Could you check a few things on this model? Use its own coordinates, in mm. Face numbers are marked on the shaded views. Round coordinates to 2 decimals unless told otherwise and drop trailing zeros. Loops run counter-clockwise (first coordinate to the right, second up) from the corner with the lowest first, then second, coordinate; pieces in that order, holes last. Notation, with made-up numbers: (12.5, -7) -> (41.5, -7) arc R13 ccw to (41.5, 10) -> close; hole circle Ø7 at (55, 39). An arc over 180 degrees is marked (long way). Use CSV: the item, a comma, the result in double quotes. Start each with the question number.
```python
from build123d import *

# Parameters (mm, degrees)
F0_W     = 25.4
F0_H     = 38.1
F0_R     = 6.35
F1_DEPTH = 133.35
F2_SIZE  = 7.62
F3_SIZE  = 7.62
F4_SIZE  = 7.62
F5_SIZE  = 7.62


with BuildPart() as f1:
    # F0 (on Front) → F1 (new body, symmetric)
    with BuildSketch(Plane.XZ):
        Rectangle(F0_W, F0_H)
        with Locations((0, 9.525)):
            Circle(F0_R, mode=Mode.SUBTRACT)
    extrude(amount=F1_DEPTH, both=True)

    # F2
    f2_edges = [f1.edges().sort_by_distance(p)[0] for p in [
        (12.7, 0, 19.05),
    ]]
    chamfer(f2_edges, length=F2_SIZE)

    # F3
    f3_edges = [f1.edges().sort_by_distance(p)[0] for p in [
        (-12.7, 0, 19.05),
    ]]
    chamfer(f3_edges, length=F3_SIZE)

    # F4
    f4_edges = [f1.edges().sort_by_distance(p)[0] for p in [
        (-12.7, 0, -19.05),
    ]]
    chamfer(f4_edges, length=F4_SIZE)

    # F5
    f5_edges = [f1.edges().sort_by_distance(p)[0] for p in [
        (12.7, 0, -19.05),
    ]]
    chamfer(f5_edges, length=F5_SIZE)


solid = f1.part
```
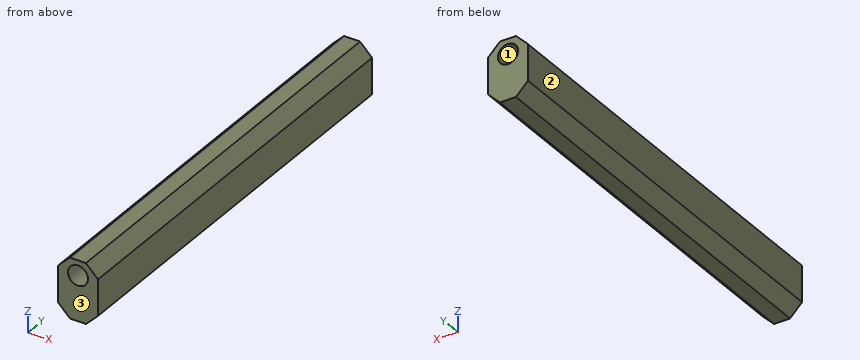
1. Suppose I cut it at D-D (z = -15). List the corners of the cut face in (x, y) for me, then the cut area to 3 significant figures.
2. Will these pins go through, and if not, where does the flat tip stop? pin 1 (8 mm diameter, centred on x = -5.5, y = 59.5, fed in from +Z); pin 2 (2 mm diameter, centred on x = 9, y = -49, fed in from +Z); pin 3 (1 mm diameter, centred on x = -7, y = 23, fed in from -Z).
3. Suppose I cut it at B-B (y = 65.5). List the corners of the cut face in (x, z) for me (3 decimals).
4. Suppose I cut it at C-C (z = 7). List the corners of the cut face in (x, y) for me.
5. We'd pull the mould along X, two halves only. Please class the marked faces 1, 2 and 3: pulls with the +X half, pulls with the -X half, needs draft (parallel to the pull), parting line crosses it, or undercut.
6. Suppose I cut it at A-A (x = 0). List the corners of the cut face in (y, z) for me (3 decimals), then the cut area to 3 significant figures.
7. If I drill on L1, parallel to X at y = 120, z = 10; L2, parallel to Z at x = -1.25, y = 23.5; L3, parallel to Z at x = 0, y = -39.5 (3 decimals), over which ranges is the centre line in solid material (lowest first)?
Geometry check:
1,outline,"(-9.13, -133.35) -> (9.13, -133.35) -> (9.13, 133.35) -> (-9.13, 133.35) -> close"
1,area,"4,870 mm²"
2,pin 1,"stops at z = 19.05"
2,pin 2,"stops at z = 16.13"
2,pin 3,"stops at z = -17.63"
3,outline,"(-12.7, -11.43) -> (-5.08, -19.05) -> (5.08, -19.05) -> (12.7, -11.43) -> (12.7, 11.43) -> (5.08, 19.05) -> (-5.08, 19.05) -> (-12.7, 11.43) -> close; hole circle Ø12.7 at (0, 9.525)"
4,outline,"(-12.7, -133.35) -> (-5.83, -133.35) -> (-5.83, 133.35) -> (-12.7, 133.35) -> close; (5.83, -133.35) -> (12.7, -133.35) -> (12.7, 133.35) -> (5.83, 133.35) -> close"
5,face 1,"undercut"
5,face 2,"pulls with the -X half"
5,face 3,"needs draft"
6,outline,"(-133.35, -19.05) -> (133.35, -19.05) -> (133.35, 3.175) -> (-133.35, 3.175) -> close; (-133.35, 15.875) -> (133.35, 15.875) -> (133.35, 19.05) -> (-133.35, 19.05) -> close"
6,area,"6,770 mm²"
7,L1,"x = -12.7 to -6.33, 6.33 to 12.7"
7,L2,"z = -19.05 to 3.3, 15.75 to 19.05"
7,L3,"z = -19.05 to 3.175, 15.875 to 19.05"
